For this review, use the dimensioned drawing (mm, ordinates from the lowest corner) and the shaded views. Give positions to 0.01 mm unless a question says otherwise; leave off trailing zeros. Order: outer loops, then holes, each group sorted by start corner. A loop starts at its lowest first (then second) coordinate and runs counter-clockwise, first axis right, second up. Notation, with made-up numbers: (-19, 0.5) - (28, 0.5) arc R17 ccw to (28, 10.5) - close; hole circle Ø10 at (-22.5, 16.25). An arc over 180 degrees is marked (long way). Answer as CSV lines item,"result". Start each with the question number.
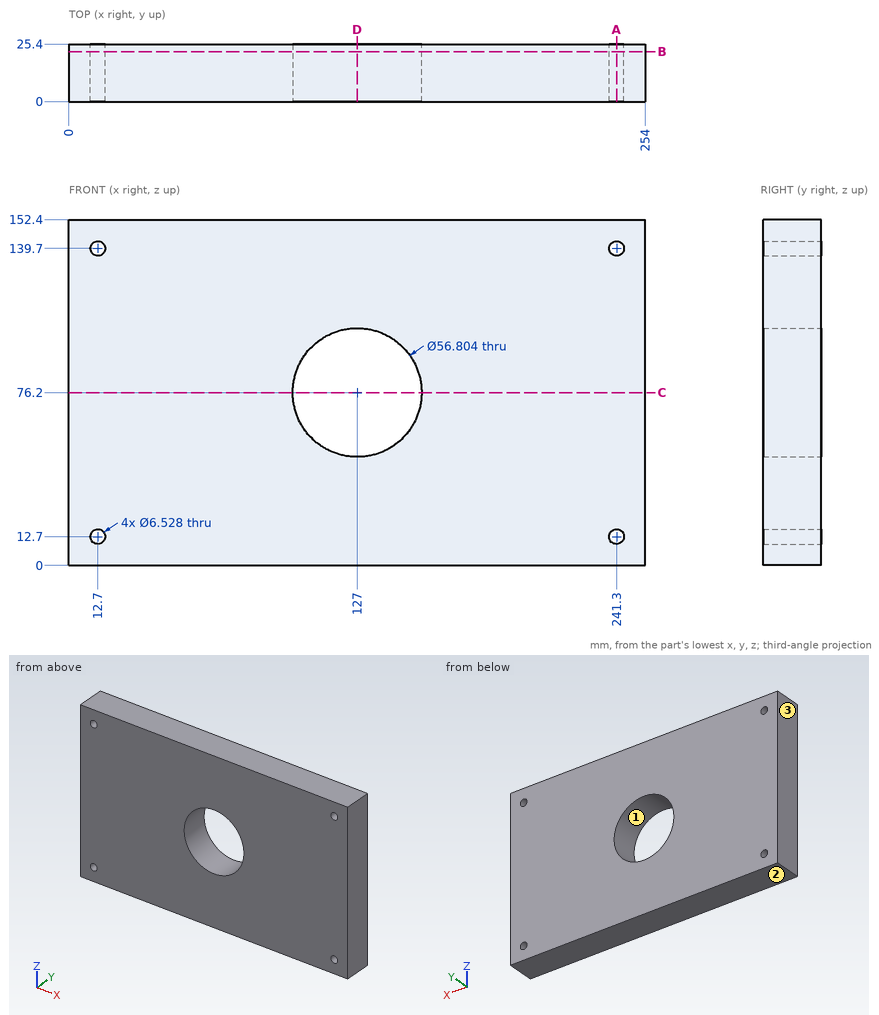
Item 1: For line 1 along Z through (x, y) = (12.7, 5.5); line 2 along X through (y, z) = (10, 66); line 3 along X through (y, z) = (14.25, 85), list the stretches that pass through material, from the lowest coordinate up.
Item 2: Take a section at D-D on x = 127. Write out the cut boundary in (y, z).
Item 3: Take a section at C-C on z = 76.2. Write out the cut boundary in (x, y).
Item 4: Take a section at A-A on x = 241.3. Write out the cut boundary in (y, z), and give its area (3 significant figures).
Item 5: Take a section at B-B on y = 22. Write out the cut boundary in (x, z).
Item 6: Mouldability with a two-part tool opening along Z and no side actions: class the marked faces 1, 2 and 3 as released by +Z, released by -Z, zero draft, split by the parting line, or undercut.
Item 7: Clearance check with a flat-ended pin moving along its axis: pin 1 (8.5 mm diameter, centred on x = 12.7, z = 12.7, fed in from -Y). State where the tip first meets the part, or that it passes through.
Data:
1,line 1,"z = 0 to 9.44, 15.96 to 136.44, 142.96 to 152.4"
1,line 2,"x = 0 to 100.49, 153.51 to 254"
1,line 3,"x = 0 to 100, 154 to 254"
2,outline,"(0, 0) - (25.4, 0) - (25.4, 47.8) - (0, 47.8) - close; (0, 104.6) - (25.4, 104.6) - (25.4, 152.4) - (0, 152.4) - close"
3,outline,"(0, 0) - (98.6, 0) - (98.6, 25.4) - (0, 25.4) - close; (155.4, 0) - (254, 0) - (254, 25.4) - (155.4, 25.4) - close"
4,outline,"(0, 0) - (25.4, 0) - (25.4, 9.44) - (0, 9.44) - close; (0, 15.96) - (25.4, 15.96) - (25.4, 136.44) - (0, 136.44) - close; (0, 142.96) - (25.4, 142.96) - (25.4, 152.4) - (0, 152.4) - close"
4,area,"3,540 mm^2"
5,outline,"(0, 0) - (254, 0) - (254, 152.4) - (0, 152.4) - close; hole circle Ø6.53 at (12.7, 12.7); hole circle Ø6.53 at (12.7, 139.7); hole circle Ø56.8 at (127, 76.2); hole circle Ø6.53 at (241.3, 12.7); hole circle Ø6.53 at (241.3, 139.7)"
6,face 1,"undercut"
6,face 2,"released by -Z"
6,face 3,"zero draft"
7,pin 1,"stops at y = 0"
